Verification items for the finished model (mm, model axes). Face numbers are marked on the shaded views. A direction names the side the tool comes from. Coordinates: 2 decimals unless noted, no trailing zeros. Write each loop counter-clockwise with the first axis right and the second up, starting at its lowest first coordinate (ties: lowest second). Pieces come first, ordered by that corner, then holes. Notation, with made-up numbers: M -34,62.5 L -22,62.5 A7 cw -22,72.5 Z; hole C 51.5,52 d7. An arc over 180 degrees is marked long. One line per item, written item: value.
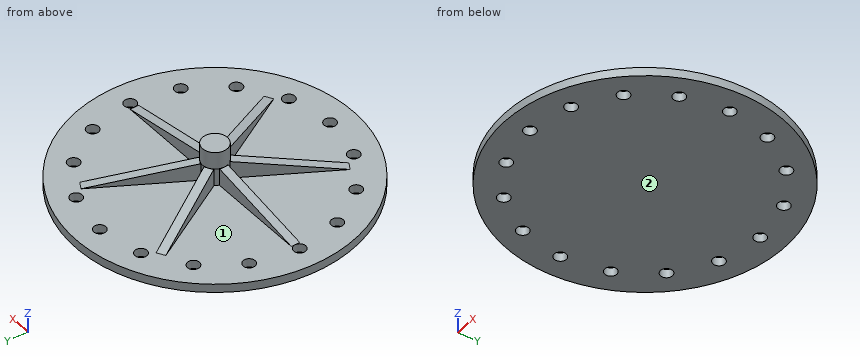
```python
from build123d import *

# Parameters (mm, degrees)
SKETCH1_R           = 162.5
BOSS_EXTRUDE1_DEPTH = 10
SKETCH2_R           = 7
CUT_EXTRUDE1_DEPTH  = 231.027172308
CIRPATTERN1_COUNT   = 16
SKETCH3_R           = 14.5
BOSS_EXTRUDE2_DEPTH = 20
RIB1_START          = -5
RIB1_DEPTH          = 10
CIRPATTERN2_COUNT   = 6
SKETCH6_R           = 14.5
BOSS_EXTRUDE3_DEPTH = 20


with BuildPart() as part:
    # Sketch1 → Boss-Extrude1 (new body)
    with BuildSketch(Plane.XY):
        Circle(SKETCH1_R)
    extrude(amount=BOSS_EXTRUDE1_DEPTH)

    # Sketch2 → Cut-Extrude1 (cut, through all)
    with BuildSketch(Plane.XY.offset(10)):
        with Locations((-51.315180135, 124.866938329)):
            Circle(SKETCH2_R)
    cut_extrude1 = extrude(amount=-CUT_EXTRUDE1_DEPTH, mode=Mode.SUBTRACT)

    # CirPattern1: Cut-Extrude1 ×16 about axis
    cirpattern1_axis = Axis((0, 0, 0), (0, 0, 1))
    for i in range(1, CIRPATTERN1_COUNT):
        add(cut_extrude1.rotate(cirpattern1_axis, i * 360 / CIRPATTERN1_COUNT), mode=Mode.SUBTRACT)

    # Sketch3 → Boss-Extrude2 (add)
    with BuildSketch(Plane.XY.offset(10)):
        Circle(SKETCH3_R)
    extrude(amount=BOSS_EXTRUDE2_DEPTH)

    # Rib1: read off the stored shape, not the designer's step
    # Rib1 outline → Rib1 (add)
    with BuildSketch(Plane(origin=(0, 0, 0), x_dir=(1, 0, 0), z_dir=(0, 1, 0)).offset(RIB1_START)):
        Polygon((-14.5, -30), (-13.610657589, -30), (-13.610657589, -10), (-127.925636392, -10), align=None)
    rib1 = extrude(amount=RIB1_DEPTH)

    # CirPattern2: Rib1 ×6 about axis
    cirpattern2_axis = Axis((0, 0, 0), (0, 0, 1))
    for i in range(1, CIRPATTERN2_COUNT):
        add(rib1.rotate(cirpattern2_axis, i * 360 / CIRPATTERN2_COUNT))

    # Sketch6 → Boss-Extrude3 (add)
    with BuildSketch(Plane.XY.offset(30)):
        Circle(SKETCH6_R)
    extrude(amount=BOSS_EXTRUDE3_DEPTH)


solid = part.part
```
Item 1: Cross-section at B-B, the plane x = 23. Enter the section's corners in (y, z), and give its area (3 significant figures).
The answers:
outline: M -160.86,0 L 160.86,0 L 160.86,10 L 49.84,10 L 49.84,22.92 L 29.84,25.97 L 29.84,10 L 5,10 L 5,28.5 L -5,28.5 L -5,10 L -29.84,10 L -29.84,25.97 L -49.84,22.92 L -49.84,10 L -160.86,10 Z
area: 3,980 mm²
Item 2: Scan lines: line 1 (X direction, y = -120, z = 8.5); line 2 (Y direction, x = -24.5, z = 12.5); line 3 (Y direction, x = -140, z = 8.5). Record each from-to range of solid material in increasing order.
The answers:
line 1: x = -109.57 to -57.3, -46.71 to 46.28, 56.35 to 109.57
line 2: y = -52.44 to -32.44, -5 to 5, 32.44 to 52.44
line 3: y = -82.5 to -4.52, 5.27 to 82.5
Item 3: Cross-section at A-A, the plane z = 23. Enter the section's corners in (x, y).
The answers:
outline: M -54.2,-5 L -13.61,-5 A14.5 ccw -11.14,-9.29 L -31.43,-44.44 L -22.77,-49.44 L -2.48,-14.29 A14.5 ccw 2.48,-14.29 L 22.77,-49.44 L 31.43,-44.44 L 11.14,-9.29 A14.5 ccw 13.61,-5 L 54.2,-5 L 54.2,5 L 13.61,5 A14.5 ccw 11.14,9.29 L 31.43,44.44 L 22.77,49.44 L 2.48,14.29 A14.5 ccw -2.48,14.29 L -22.77,49.44 L -31.43,44.44 L -11.14,9.29 A14.5 ccw -13.61,5 L -54.2,5 Z
Item 4: Go/stop test with flat-tipped pins: P1, Ø12.5, axis at x = -95.19, y = 95.72, coming from the -Z side; P2, Ø1, axis at x = 10.5, y = 11, coming from the +Z side; P3, Ø1.5, axis at y = -34.5, z = 7.5, coming from the +X side; P4, Ø10, axis at x = -79.5, z = 19.5, coming from the -Y side. Record where each tip stops, or that it passes through.
The answers:
P1: passes through
P2: stops at z = 30
P3: stops at x = 158.96
P4: stops at y = -5
Item 5: Cross-section at C-C, the plane z = 46. Enter the section's corners in (x, y), and give its area (3 significant figures).
The answers:
outline: C 0,0 d29
area: 661 mm²
Item 6: Access from +Z, -Z, +X, -X, +Y, -Y to the whole of each face (thin tool, end or side, straight path). Record for the marked faces 1 and 2.
The answers:
face 1: +Z
face 2: -Z, +X, -X, +Y, -Y
